Design review of the part shown in the three views and the two pictorial views. Dimensions are in mm from the part's minimum x, y and z. A direction names the side the tool comes from. Give positions to 0.01 mm unless a question says otherwise; leave off trailing zeros. Loops run counter-clockwise (first coordinate to the right, second up) from the corner with the lowest first, then second, coordinate; pieces in that order, holes last.
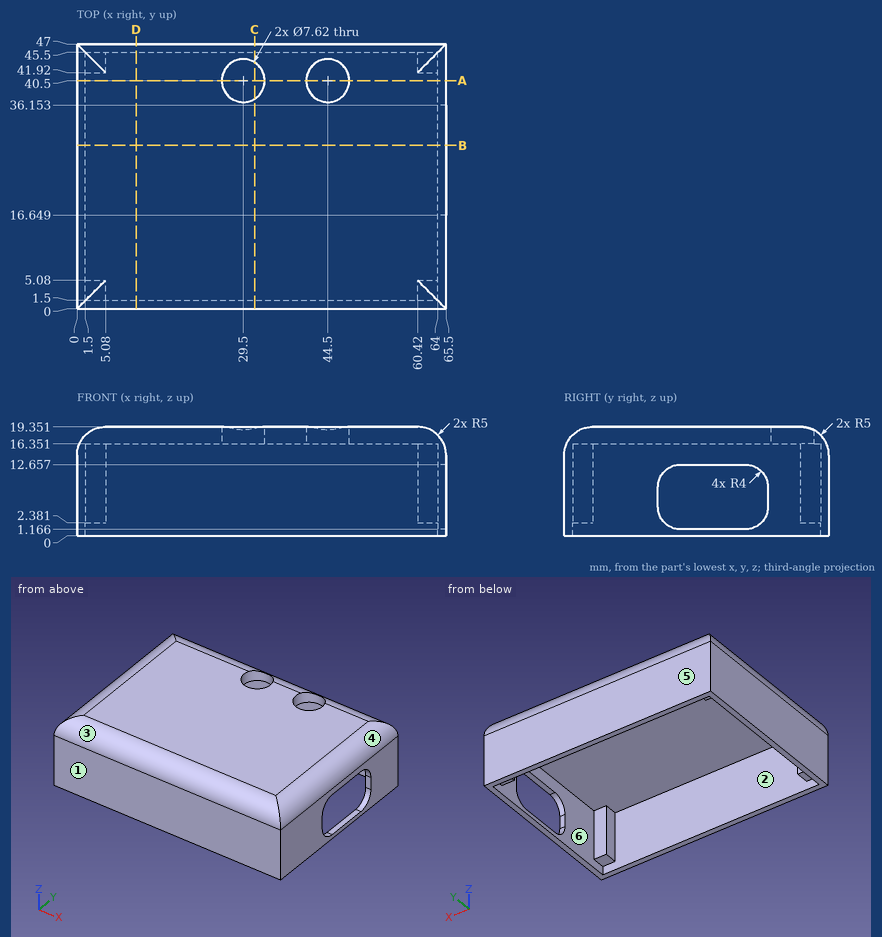
Q1. Wall thickness on line 1 (X direction, y = 4.5, z = 10.5); line 2 (X direction, y = 10, z = 12); line 3 (X direction, y = 40.5, z = 18.45) (1 decimal): over which ranges is each line inside the solid? List them lowest first.
Results:
line 1: x = 0 to 5.08, 60.42 to 65.5
line 2: x = 0 to 1.5, 64 to 65.5
line 3: x = 2.1 to 25.7, 33.3 to 40.7, 48.3 to 63.4
Q2. Take a section at C-C (x = 31.5). Give the boundary of the cut face in (y, z).
Results:
outline: (0, 0) - (1.5, 0) - (1.5, 16.35) - (37.26, 16.35) - (37.26, 19.35) - (5, 19.35) arc R5 ccw to (0, 14.35) - close; (43.74, 16.35) - (45.5, 16.35) - (45.5, 0) - (47, 0) - (47, 14.35) arc R5 ccw to (43.74, 19.04) - close
Q3. Insertion check: pin 1 (1.5 mm diameter, centred on y = 22.5, z = 16, fed in from +X); pin 2 (1.8 mm diameter, centred on x = 62, y = 3, fed in from -Z). Each pin has a flat end and moves straight along its axis. Give the tip position at first contact, or say it passes through.
Results:
pin 1: stops at x = 65.42
pin 2: stops at z = 2.38
Q4. Draft analysis for pull direction Y (two halves, no side actions). For the marked faces 3, 4, 5 and 6, state which applies: pulls with the +Y half, pulls with the -Y half, needs draft (parallel to the pull), parting line crosses it, or undercut.
Results:
face 3: pulls with the -Y half
face 4: needs draft
face 5: pulls with the +Y half
face 6: undercut
Q5. Take a section at D-D (x = 10.5). Give the boundary of the cut face in (y, z).
Results:
outline: (0, 0) - (1.5, 0) - (1.5, 16.35) - (45.5, 16.35) - (45.5, 0) - (47, 0) - (47, 14.35) arc R5 ccw to (42, 19.35) - (5, 19.35) arc R5 ccw to (0, 14.35) - close
Q6. Take a section at A-A (y = 40.5). Give the boundary of the cut face in (x, z), plus the area to 3 significant figures.
Results:
outline: (0, 0) - (1.5, 0) - (1.5, 16.35) - (25.69, 16.35) - (25.69, 19.35) - (5, 19.35) arc R5 ccw to (0, 14.35) - close; (33.31, 16.35) - (40.69, 16.35) - (40.69, 19.35) - (33.31, 19.35) - close; (48.31, 16.35) - (64, 16.35) - (64, 0) - (65.5, 0) - (65.5, 14.35) arc R5 ccw to (60.5, 19.35) - (48.31, 19.35) - close
area: 189 mm2
Q7. Take a section at B-B (y = 29). Give the boundary of the cut face in (x, z).
Results:
outline: (0, 0) - (1.5, 0) - (1.5, 16.35) - (64, 16.35) - (64, 12.66) - (65.5, 12.66) - (65.5, 14.35) arc R5 ccw to (60.5, 19.35) - (5, 19.35) arc R5 ccw to (0, 14.35) - close; (64, 0) - (65.5, 0) - (65.5, 1.17) - (64, 1.17) - close
Q8. Tool access review of the marked faces 1 and 2: name each direction out of +Z, -Z, +X, -X, +Y, -Y from which nothing blocks a thin tool from reaching the whole face with its end or side.
Results:
face 1: +Z, -Z, +X, -X, -Y
face 2: -Z
